Autodesk Inventor part; units mm, degrees
ref_plane "YZ Plane" through (0, 0, 0) normal (1, 0, 0) x (0, 1, 0)
ref_plane "XZ Plane" through (0, 0, 0) normal (0, 1, 0) x (-1, 0, 0)
ref_plane "XY Plane" through (0, 0, 0) normal (0, 0, 1) x (1, 0, 0)
sketch "Sketch1" plane through (0, 0, 0) normal (0, 0, 1) x (1, 0, 0)
  line L0 (0, 0) -> (190, 0)
  line L1 (190, 0) -> (190, 35)
  line L2 (190, 35) -> (0, 35)
  line L3 (0, 35) -> (0, 0)
  circle A0 centre (7.5, 17.5) radius 1.5
  circle A1 centre (182.5, 17.5) radius 1.5
  point P0 (0, 17.5)
  dimension "d0" = 190
  dimension "d1" = 35
  dimension "d2" = 3
  dimension "d3" = 7.5
  dimension "d4" = 3
  dimension "d5" = 7.5
extrude "Extrusion1" add sketch "Sketch1" along normal blind 5
sketch "Sketch2" plane through (0, 0, 0) normal (0, 0, -1) x (-1, 0, 0)
  line L0 (0, 0) -> (-190, 0)
  line L1 (-190, 35) -> (0, 35)
  line L2 (-15.5, 0) -> (-174.5, 0)
  line L3 (-174.5, 0) -> (-174.5, 35)
  line L4 (-174.5, 35) -> (-15.5, 35)
  line L5 (-15.5, 35) -> (-15.5, 0)
  point P0 (-95, 0)
  dimension "d8" = 159
extrude "Extrusion2" add sketch "Sketch2" along normal blind 5
sketch "Sketch3" plane through (0, 0, 5) normal (0, 0, 1) x (1, 0, 0)
  circle A0 centre (182.5, 17.5) radius 1.5
  circle A1 centre (7.5, 17.5) radius 1.5
  line L0 (0, 0) -> (190, 0)
  line L1 (190, 0) -> (190, 35)
  line L2 (190, 35) -> (0, 35)
  line L3 (0, 35) -> (0, 0)
  line L4 (1, 34) -> (189, 34)
  line L5 (189, 34) -> (189, 1)
  line L6 (189, 1) -> (1, 1)
  line L7 (1, 1) -> (1, 34)
  dimension "d11" = 1
extrude "Extrusion3" cut sketch "Sketch3" against normal through all contours L3 L2 L1 L0
sketch "Sketch4" plane through (0, 0, 5) normal (0, 0, 1) x (1, 0, 0)
  line L0 (39.5, 27.5) -> (69.5, 27.5)
  line L1 (69.5, 27.5) -> (69.5, 7.5)
  line L2 (69.5, 7.5) -> (39.5, 7.5)
  line L3 (39.5, 7.5) -> (39.5, 27.5)
  line L4 (84.5, 27.5) -> (114.5, 27.5)
  line L5 (114.5, 27.5) -> (114.5, 7.5)
  line L6 (114.5, 7.5) -> (84.5, 7.5)
  line L7 (84.5, 7.5) -> (84.5, 27.5)
  line L8 (129.5, 27.5) -> (150.5, 27.5)
  line L9 (150.5, 27.5) -> (150.5, 7.5)
  line L10 (150.5, 7.5) -> (129.5, 7.5)
  line L11 (129.5, 7.5) -> (129.5, 27.5)
  line L12 (39.5, 17.5) -> (150.5, 17.5) construction
  line L13 (189, 34) -> (1, 34)
  circle A0 centre (7.5, 17.5) radius 1.5
  point P0 (0, 0)
  point P1 (95, 17.5)
  point P2 (95, 34)
  point P3 (114.5, 17.5)
  dimension "d14" = 30
  dimension "d15" = 20
  dimension "d16" = 30
  dimension "d17" = 20
  dimension "d18" = 21
  dimension "d19" = 20
  dimension "d20" = 15
  dimension "d21" = 15
extrude "Extrusion4" cut sketch "Sketch4" against normal through all contours L0 L1 L2 L3 | L4 L5 L6 L7 | L8 L9 L10 L11
sketch "Sketch5" plane through (0, 0, 5) normal (0, 0, 1) x (1, 0, 0)
  line L0 (39.5, 27.5) -> (39.5, 7.5)
  line L1 (39.5, 7.5) -> (69.5, 7.5)
  line L2 (69.5, 7.5) -> (69.5, 27.5)
  line L3 (69.5, 27.5) -> (39.5, 27.5)
  line L4 (129.5, 27.5) -> (129.5, 7.5)
  line L5 (129.5, 7.5) -> (150.5, 7.5)
  line L6 (150.5, 7.5) -> (150.5, 27.5)
  line L7 (150.5, 27.5) -> (129.5, 27.5)
  line L8 (84.5, 27.5) -> (84.5, 7.5)
  line L9 (84.5, 7.5) -> (114.5, 7.5)
  line L10 (114.5, 7.5) -> (114.5, 27.5)
  line L11 (114.5, 27.5) -> (84.5, 27.5)
  line L12 (174.5, 1) -> (15.5, 1)
  line L13 (15.5, 1) -> (15.5, 34)
  line L14 (15.5, 34) -> (174.5, 34)
  line L15 (174.5, 34) -> (174.5, 1)
  point P0 (0, 0)
extrude "Extrusion5" add sketch "Sketch5" along normal blind 25
sketch "Sketch6" plane through (0, 0, -5) normal (0, 0, -1) x (-1, 0, 0)
  line L0 (-69.5, 27.5) -> (-39.5, 27.5)
  line L1 (-39.5, 27.5) -> (-39.5, 7.5)
  line L2 (-69.5, 7.5) -> (-69.5, 27.5)
  line L3 (-84.5, 27.5) -> (-84.5, 7.5)
  line L4 (-114.5, 27.5) -> (-84.5, 27.5)
  line L5 (-114.5, 7.5) -> (-114.5, 27.5)
  line L6 (-39.5, 25) -> (-34.5, 25)
  line L7 (-34.5, 25) -> (-34.5, 10)
  line L8 (-34.5, 10) -> (-39.5, 10)
  line L9 (-39.5, 10) -> (-39.5, 25)
  line L10 (-69.5, 25) -> (-74.5, 25)
  line L11 (-74.5, 25) -> (-74.5, 10)
  line L12 (-74.5, 10) -> (-69.5, 10)
  line L13 (-69.5, 10) -> (-69.5, 25)
  line L14 (-84.5, 25) -> (-79.5, 25)
  line L15 (-79.5, 25) -> (-79.5, 10)
  line L16 (-79.5, 10) -> (-84.5, 10)
  line L17 (-84.5, 10) -> (-84.5, 25)
  line L18 (-114.5, 25) -> (-119.5, 25)
  line L19 (-119.5, 25) -> (-119.5, 10)
  line L20 (-119.5, 10) -> (-114.5, 10)
  line L21 (-114.5, 10) -> (-114.5, 25)
  point P0 (0, 0)
  point P1 (-39.5, 17.5)
  dimension "d26" = 15
  dimension "d27" = 5
  dimension "d28" = 5
  dimension "d29" = 5
  dimension "d30" = 5
extrude "Extrusion6" cut sketch "Sketch6" against normal blind 22
properties part number "BP011" material "ABS Plastic"
Source: CAD feature listing. Evaluate the final solid. Frame: model axes, mm. A direction names the side the tool comes from. Round coordinates to 2 decimals unless told otherwise and drop trailing zeros. Write each loop counter-clockwise with the first axis right and the second up, starting at its lowest first coordinate (ties: lowest second). Pieces come first, ordered by that corner, then holes. Notation, with made-up numbers: (-28, 25.25) - (-8, 25.25) arc R29 cw to (-8, 59.25) - close; hole circle Ø1 at (23, -7.75). An arc over 180 degrees is marked (long way). Use CSV: the item, a comma, the result in double quotes. Start each with the question number.
(1) First-contact query: pin 1 Ø4.5 at (x, y) = (9, 18.5) entering from +Z; pin 2 Ø7 at (x, y) = (178.5, 15) entering from -Z; pin 3 Ø6 at (y, z) = (18.5, 9) entering from +X; pin 4 Ø1 at (x, y) = (67.5, 17.5) entering from -Z. Flat tips, straight axial feed; report the tip coordinate or a pass-through.
(2) Set-up query: faces 4 (the face through (10, 18, 5)), 5 (the face through (69.5, 17, 20)), 6 (the face through (119.5, 18, 6)), 7 (the face through (174.5, 17, -2)). Return all of +Z, -Z, +X, -X, +Y, -Y with unobstructed straight access to the full face (end or side cutting, diameter ignored); none if empty.
(3) Cut plane C-C, the plane z = 27. Return loops of the section in (x, y), and give its area (3 significant figures).
(4) Mould query, pull axis Y, two halves, no side actions, for faces 1 (the face through (55, 27.5, 12)), 2 (the face through (96, 1, 12)), 3 (the face through (15.5, 18, -2)). Classes: pulls with the +Y half, pulls with the -Y half, needs draft (parallel to the pull), parting line crosses it, or undercut.
(5) Cut plane B-B, the plane z = 3. Give the number of separate pieces and of enclosed holes in the cut face, and give its area (3 significant figures).
(6) Material intervals for probe 1 along X at (y, z) = (23.5, 15); probe 2 along Y at (x, z) = (182.5, 2.3); probe 3 along Y at (x, z) = (147, 23), sorted ascending. Write a range as [from, to].
(7) Cut plane A-A, the plane x = 105. Return loops of the section in (y, z), and give its area (3 significant figures).
Geometry says:
1,pin 1,"z = 5"
1,pin 2,"z = 0"
1,pin 3,"x = 174.5"
1,pin 4,"through"
2,face 4,"+Z, -X, +Y, -Y"
2,face 5,"+Z, -Z"
2,face 6,"-Z"
2,face 7,"-Z, +X, +Y, -Y"
3,outline,"(15.5, 1) - (174.5, 1) - (174.5, 34) - (15.5, 34) - close; hole (39.5, 7.5) - (69.5, 7.5) - (69.5, 27.5) - (39.5, 27.5) - close; hole (84.5, 7.5) - (114.5, 7.5) - (114.5, 27.5) - (84.5, 27.5) - close; hole (129.5, 7.5) - (150.5, 7.5) - (150.5, 27.5) - (129.5, 27.5) - close"
3,area,"3,630 mm²"
4,face 1,"undercut"
4,face 2,"pulls with the -Y half"
4,face 3,"needs draft"
5,separate pieces,"1"
5,enclosed holes,"5"
5,area,"4,270 mm²"
6,probe 1,"[15.5, 34.5], [74.5, 79.5], [119.5, 129.5], [150.5, 174.5]"
6,probe 2,"[1, 16], [19, 34]"
6,probe 3,"[1, 7.5], [27.5, 34]"
7,outline,"(1, -5) - (7.5, -5) - (7.5, 30) - (1, 30) - close; (27.5, -5) - (34, -5) - (34, 30) - (27.5, 30) - close"
7,area,"455 mm²"
